```python
from build123d import *

# Parameters (mm, degrees)
F0_R      = 9.817303
F1_DEPTH  = 25.4
F3_R      = 6.778938
F4_DEPTH  = 25.4
F5_R      = 14.680473
F6_DEPTH  = 7.112
F7_R      = 9.730781
F8_DEPTH  = 25.4
F9_R      = 6.676703
F10_DEPTH = 92.456
F11_D     = 13.55852


with BuildPart() as f1:
    # F0 (on Top) → F1 (new body)
    with BuildSketch(Plane.XY):
        Circle(F0_R)
    extrude(amount=F1_DEPTH)

    # F3 (on face) → F4 (cut)
    with BuildSketch(Plane.XY.offset(25.4)):
        Circle(F3_R)
    extrude(amount=-F4_DEPTH, mode=Mode.SUBTRACT)

    # F5 (on Top) → F6 (join)
    with BuildSketch(Plane.XY):
        Circle(F5_R)
    extrude(amount=-F6_DEPTH)

    # F7 (on face) → F8 (join)
    with BuildSketch(Plane(origin=(0, 0, -7.112), x_dir=(1, 0, 0), z_dir=(0, 0, -1))):
        Circle(F7_R)
    extrude(amount=F8_DEPTH)

    # F9 (on face) → F10 (join)
    with BuildSketch(Plane(origin=(0, 0, -32.512), x_dir=(1, 0, 0), z_dir=(0, 0, -1))):
        Circle(F9_R)
    extrude(amount=-F10_DEPTH)

    # F11 (through all)
    with Locations(Plane(origin=(0, 0, -32.512), x_dir=(1, 0, 0), z_dir=(0, 0, -1))):
        with Locations((0, 0)):
            Hole(F11_D / 2)


solid = f1.part
```
Model file for the job. Use its own axes, mm. A direction names the side the tool comes from. Round coordinates to 2 decimals unless told otherwise and drop trailing zeros. Write each loop counter-clockwise with the first axis right and the second up, starting at its lowest first coordinate (ties: lowest second). Pieces come first, ordered by that corner, then holes. Notation, with made-up numbers: (58, 6) -> (104, 6) arc R20 cw to (104, 20) -> close; hole circle Ø9 at (15.25, -7.5). An arc over 180 degrees is marked (long way). Answer as CSV lines item,"result".
1. Pin check, flat tips, straight feed: pin 1 Ø5 at (x, z) = (3.5, 11.5) entering from +Y; pin 2 Ø3 at (y, z) = (10.5, -24) entering from -X; pin 3 Ø1.5 at (y, z) = (-2, -14.5) entering from -X; pin 4 Ø17.5 at (x, y) = (0, 0) entering from +Z. Stop position of each tip, or through.
Resolved:
pin 1,"y = 9.77"
pin 2,"x = -3.7"
pin 3,"x = -9.65"
pin 4,"z = 25.4"
2. Mould opens along Y. For faces 4 (the face through (-6.466, -2.036, -3.151)), 5 (the face through (-3.18, -14.33, -3.51)), 6 (the face through (3, -10, 0)) say: +Y half, -Y half, draft (parallel to the pull), parting line (faces both ways), or undercut.
Resolved:
face 4,"undercut"
face 5,"parting line"
face 6,"draft"
3. Slice it at D-D, the plane y = -11.5. List the corners of the cut face in (x, z).
Resolved:
outline,"(-9.13, -7.11) -> (9.13, -7.11) -> (9.13, 0) -> (-9.13, 0) -> close"
4. Tool access for faces 1 (the face through (2, 7, 25.4)), 2 (the face through (-9.808, 0.432, 12.522)), 3 (the face through (3, -10, -7.112)): list every direction of +Z, -Z, +X, -X, +Y, -Y with a clear straight run to the whole face (end or side of a thin tool).
Resolved:
face 1,"+Z, +X, -X, +Y, -Y"
face 2,"+Z"
face 3,"-Z"
5. Slice it at C-C, the plane z = 10. List the corners of the cut face in (x, y).
Resolved:
outline,"circle Ø19.63 at (0, 0); hole circle Ø13.56 at (0, 0)"
6. Slice it at A-A, the plane y = 0. List the corners of the cut face in (x, z), plus the area to 3 significant figures.
Resolved:
outline,"(-14.68, -7.11) -> (-9.73, -7.11) -> (-9.73, -32.51) -> (-6.78, -32.51) -> (-6.78, 25.4) -> (-9.82, 25.4) -> (-9.82, 0) -> (-14.68, 0) -> close; (6.78, -32.51) -> (9.73, -32.51) -> (9.73, -7.11) -> (14.68, -7.11) -> (14.68, 0) -> (9.82, 0) -> (9.82, 25.4) -> (6.78, 25.4) -> close"
area,"417 mm²"
7. Drill centre lines: line 1 (Y direction, x = 0, z = 14); line 2 (Y direction, x = 0, z = -18); line 3 (Z direction, x = -1.25, y = -12.25). Where is each one in solid material? Low to high.
Resolved:
line 1,"-9.82 to -6.78, 6.78 to 9.82"
line 2,"-9.73 to -6.78, 6.78 to 9.73"
line 3,"-7.11 to 0"
